Part model, mm, in its own coordinate system. A direction names the side the tool comes from. Coordinates: 2 decimals unless noted, no trailing zeros. Loops run counter-clockwise (first coordinate to the right, second up) from the corner with the lowest first, then second, coordinate; pieces in that order, holes last. Notation, with made-up numbers: (35.25, -8.5) - (73.25, -8.5) arc R18 cw to (73.25, -4.5) - close; hole circle Ø2 at (-32, 76). An arc over 180 degrees is marked (long way). Use a Markdown table: item, result. Add a question column.
1) Band-saw the part on D-D (x = 24). Give the cut face in (y, z), plus the area to 3 significant figures.
2) Probe probe 1 along X at (y, z) = (14.5, 29.75); probe 2 along Z at (x, y) = (27, 11.5); probe 3 along Y at (x, z) = (4.5, 21.5). List the from-to ranges inside material, lowest first. Write a range as [from, to].
3) Band-saw the part on C-C (y = 6). Give the number of separate pieces and of enclosed holes in the cut face, plus the area to 3 significant figures.
4) Tool access for faces 1 (the face through (27, 11, 32)), 2 (the face through (18, 22, 20)), 3 (the face through (36.4, 11, 19)): list every direction of +Z, -Z, +X, -X, +Y, -Y with a clear straight run to the whole face (end or side of a thin tool).
5) Band-saw the part on A-A (z = 29.75). Give the cut face in (x, y).
6) Band-saw the part on B-B (x = 8.2). Give the cut face in (y, z).
7) Drop flat-ended pins along their axis: P1, Ø6, axis at x = 8.2, z = 9.75, coming from the +Y side; P2, Ø6.5, axis at x = 66.58, z = 48.66, coming from the -Y side; P3, Ø6.5, axis at y = 9.5, z = 17.5, coming from the +X side; P4, Ø1.5, axis at x = 52, y = 3.5, coming from the -Z side. Give the stop position or say it passes through.
8) Pull direction Z, two halves, no side cores. Call faces 4 (the face through (8.3, 10.8, 32.3)), 5 (the face through (31, 0, 49)), 6 (the face through (40, 12, 79.5)): +Z half, -Z half, draft (parallel to the pull), parting line (faces both ways), or undercut.
from build123d import *

# Parameters (mm, degrees)
SKETCH1_W               = 36.4
SKETCH1_H               = 39.5
SKETCH1_R               = 2.55
BOSS_EXTRUDE1_DEPTH     = 22
BOSS_EXTRUDE2_START     = -22
SKETCH2_W               = 82
SKETCH2_H               = 40
BOSS_EXTRUDE2_DEPTH     = 25
F_5_0MM_DOWEL_HOLE1_D   = 5.1
CUT_EXTRUDE1_DEPTH      = 30
CUT_EXTRUDE1_DEPTH_BACK = 50
SKETCH3_W               = 85.710853131
SKETCH3_H               = 93.141989814


with BuildPart() as part:
    # Sketch1 → Boss-Extrude1 (new body)
    with BuildSketch(Plane(origin=(0, 0, 0), x_dir=(1, 0, 0), z_dir=(0, 1, 0))):
        with Locations((18.2, 19.75)):
            Rectangle(SKETCH1_W, SKETCH1_H)
        with Locations(Location((8.2, 29.75, 0), (0, 0, 270))):
            Circle(SKETCH1_R, mode=Mode.SUBTRACT)
        with Locations(Location((28.2, 29.75, 0), (0, 0, 270))):
            Circle(SKETCH1_R, mode=Mode.SUBTRACT)
        with Locations(Location((28.2, 19.75, 0), (0, 0, 270))):
            Circle(SKETCH1_R, mode=Mode.SUBTRACT)
        with Locations(Location((28.2, 9.75, 0), (0, 0, 270))):
            Circle(SKETCH1_R, mode=Mode.SUBTRACT)
        with Locations(Location((8.2, 19.75, 0), (0, 0, 270))):
            Circle(SKETCH1_R, mode=Mode.SUBTRACT)
        with Locations(Location((8.2, 9.75, 0), (0, 0, 270))):
            Circle(SKETCH1_R, mode=Mode.SUBTRACT)
    boss_extrude1 = extrude(amount=BOSS_EXTRUDE1_DEPTH)

    # Sketch2 → Boss-Extrude2 (add)
    with BuildSketch(Plane(origin=(0, 22, 0), x_dir=(1, 0, 0), z_dir=(0, 1, 0)).offset(BOSS_EXTRUDE2_START)):
        with Locations((41, 59.5)):
            Rectangle(SKETCH2_W, SKETCH2_H)
    boss_extrude2 = extrude(amount=BOSS_EXTRUDE2_DEPTH)

    # Mirror3: Boss-Extrude1, Boss-Extrude2 across plane
    add(boss_extrude1.mirror(Plane(origin=(0, 22, 0), x_dir=(1, 0, 0), z_dir=(0, 0, -1))))
    add(boss_extrude2.mirror(Plane(origin=(0, 22, 0), x_dir=(1, 0, 0), z_dir=(0, 0, -1))))

    # Ø5.0mm Dowel Hole1 (through all)
    with Locations(Plane(origin=(42.996100309, 25, 52.24566701), x_dir=(0, 0, 1), z_dir=(0, 1, 0))):
        with Locations((0, 0), (18, 20), (-3.585786438, 23.585786437)):
            Hole(F_5_0MM_DOWEL_HOLE1_D / 2)

    # Sketch3 → Cut-Extrude1 (cut, two sides: drawn at the far end of the back side and taken through both)
    with BuildSketch(Plane(origin=(0, 22, 0), x_dir=(1, 0, 0), z_dir=(0, 1, 0)).offset(-CUT_EXTRUDE1_DEPTH_BACK)):
        with Locations((42.855426566, 46.570994907)):
            Rectangle(SKETCH3_W, SKETCH3_H)
    extrude(amount=CUT_EXTRUDE1_DEPTH + CUT_EXTRUDE1_DEPTH_BACK, mode=Mode.SUBTRACT)


solid = part.part
Answer block:
| question | item | result |
|---|---|---|
| 1 | outline | (0, 0) - (22, 0) - (22, 39.5) - (25, 39.5) - (25, 79.5) - (0, 79.5) - close |
| 1 | area | 1,870 mm2 |
| 2 | probe 1 | [0, 5.65], [10.75, 25.65], [30.75, 36.4] |
| 2 | probe 2 | [0, 7.5], [12, 17.5], [22, 27.5], [32, 79.5] |
| 2 | probe 3 | [0, 22] |
| 3 | separate pieces | 1 |
| 3 | enclosed holes | 9 |
| 3 | area | 4,530 mm2 |
| 4 | face 1 | +Y, -Y |
| 4 | face 2 | -Z, +X, -X, +Y |
| 4 | face 3 | -Z, +X, +Y, -Y |
| 5 | outline | (0, 0) - (5.65, 0) - (5.65, 22) - (0, 22) - close; (10.75, 0) - (25.65, 0) - (25.65, 22) - (10.75, 22) - close; (30.75, 0) - (36.4, 0) - (36.4, 22) - (30.75, 22) - close |
| 6 | outline | (0, 0) - (22, 0) - (22, 7.2) - (0, 7.2) - close; (0, 12.3) - (22, 12.3) - (22, 17.2) - (0, 17.2) - close; (0, 22.3) - (22, 22.3) - (22, 27.2) - (0, 27.2) - close; (0, 32.3) - (22, 32.3) - (22, 39.5) - (25, 39.5) - (25, 79.5) - (0, 79.5) - close |
| 7 | P1 | y = 22 |
| 7 | P2 | y = 0 |
| 7 | P3 | x = 36.4 |
| 7 | P4 | z = 39.5 |
| 8 | face 4 | undercut |
| 8 | face 5 | draft |
| 8 | face 6 | +Z half |
